```python
from build123d import *

# Parameters (mm, degrees)
BOSS_EXTRUDE1_DEPTH = 3
SKETCH4_W           = 10.2
SKETCH4_H           = 3.2
SKETCH4_W_2         = 3.2
SKETCH4_H_2         = 10.2
SKETCH4_W_3         = 29.422217102
SKETCH4_H_3         = 12.077782898
CUT_EXTRUDE1_DEPTH  = 4


with BuildPart() as part:
    # Sketch1 → Boss-Extrude1 (new body)
    with BuildSketch(Plane(origin=(0, 0, 0), x_dir=(1, 0, 0), z_dir=(0, 1, 0))):
        Polygon((129.394434203, 22.05), (22.05, 22.05), (22.05, 110.344434203), (0, 110.344434203), (0, 0), (129.394434203, 0), align=None)
    extrude(amount=-BOSS_EXTRUDE1_DEPTH)

    # Sketch4 → Cut-Extrude1 (cut, through all)
    with BuildSketch(Plane(origin=(0, 0, 0), x_dir=(1, 0, 0), z_dir=(0, 1, 0))):
        with Locations((54.222217102, 20.55)):
            Rectangle(SKETCH4_W, SKETCH4_H)
        with Locations((74.222217102, 20.55)):
            Rectangle(SKETCH4_W, SKETCH4_H)
        with Locations((114.222217102, 1.5)):
            Rectangle(SKETCH4_W, SKETCH4_H)
        with Locations((1.5, 15.172217102)):
            Rectangle(SKETCH4_W_2, SKETCH4_H_2)
        with Locations((34.222217102, 20.55)):
            Rectangle(SKETCH4_W, SKETCH4_H)
        with Locations((24.611108551, 1.5)):
            Rectangle(SKETCH4_W_3, SKETCH4_H)
        with Locations((32.35, 9.6)):
            Rectangle(SKETCH4_W, SKETCH4_H)
        with Locations((54.222217102, 1.5)):
            Rectangle(SKETCH4_W, SKETCH4_H)
        with Locations((74.222217102, 1.5)):
            Rectangle(SKETCH4_W, SKETCH4_H)
        with Locations((9.6, 15.172217102)):
            Rectangle(SKETCH4_W_2, SKETCH4_H_2)
        with Locations((1.5, 35.172217102)):
            Rectangle(SKETCH4_W_2, SKETCH4_H_2)
        with Locations((9.6, 35.172217102)):
            Rectangle(SKETCH4_W_2, SKETCH4_H_2)
        with Locations((20.55, 35.172217102)):
            Rectangle(SKETCH4_W_2, SKETCH4_H_2)
        with Locations((1.5, 108.844434203)):
            Rectangle(SKETCH4_W_2, SKETCH4_H)
        with Locations((9.6, 108.844434203)):
            Rectangle(SKETCH4_W_2, SKETCH4_H)
        with Locations((9.6, 95.172217102)):
            Rectangle(SKETCH4_W_2, SKETCH4_H_2)
        with Locations((1.5, 95.172217102)):
            Rectangle(SKETCH4_W_2, SKETCH4_H_2)
        with Locations((1.5, 75.172217102)):
            Rectangle(SKETCH4_W_2, SKETCH4_H_2)
        with Locations((9.6, 75.172217102)):
            Rectangle(SKETCH4_W_2, SKETCH4_H_2)
        with Locations((20.55, 95.172217102)):
            Rectangle(SKETCH4_W_2, SKETCH4_H_2)
        with Locations((20.55, 75.172217102)):
            Rectangle(SKETCH4_W_2, SKETCH4_H_2)
        with Locations((1.5, 55.172217102)):
            Rectangle(SKETCH4_W_2, SKETCH4_H_2)
        with Locations((9.6, 55.172217102)):
            Rectangle(SKETCH4_W_2, SKETCH4_H_2)
        with Locations((20.55, 55.172217102)):
            Rectangle(SKETCH4_W_2, SKETCH4_H_2)
        with Locations((127.894434203, 16.111108551)):
            Rectangle(SKETCH4_W_2, SKETCH4_H_3)
        with Locations((94.222217102, 1.5)):
            Rectangle(SKETCH4_W, SKETCH4_H)
        with Locations((114.222217102, 20.55)):
            Rectangle(SKETCH4_W, SKETCH4_H)
        with Locations((94.222217102, 20.55)):
            Rectangle(SKETCH4_W, SKETCH4_H)
        with Locations((116.094434203, 9.6)):
            Rectangle(SKETCH4_W, SKETCH4_H)
    extrude(amount=-CUT_EXTRUDE1_DEPTH, mode=Mode.SUBTRACT)


solid = part.part
```
Can you work these out from the model? Positions are in its coordinate system, mm. A direction names the side the tool comes from. Give positions to 0.01 mm unless a question says otherwise; leave off trailing zeros. Loops run counter-clockwise (first coordinate to the right, second up) from the corner with the lowest first, then second, coordinate; pieces in that order, holes last. Notation, with made-up numbers: M 48.5,12.25 L 54.5,12.25 A8 cw 54.5,16.25 Z; hole C 58,-2 d11. An arc over 180 degrees is marked long. One line per item, written item: value.
(1) We'd pull the mould along X, two halves only. Please class faces 1 (the face through (22.05, -1, -85)), 2 (the face through (9.9, -1, -2)), 3 (the face through (2, -1, -90.072)): released by +X, released by -X, zero draft, split by the parting line, or undercut.
Returned:
face 1: released by +X
face 2: undercut
face 3: zero draft
(2) Suppose I cut it at C-C on y = -1.25. Count the separate pieces of the cut face and the enclosed holes in it, plus the area to 3 significant figures.
Returned:
separate pieces: 1
enclosed holes: 7
area: 3,850 mm^2
(3) Will these pins go through, and if not, where does the flat tip stop? pin 1 (0.9 mm diameter, centred on y = -1, z = -54, fed in from +X); pin 2 (1.5 mm diameter, centred on x = 1.5, y = -1, fed in from -Z); pin 3 (0.9 mm diameter, centred on y = -1, z = -20, fed in from +X).
Returned:
pin 1: x = 18.95
pin 2: z = -107.24
pin 3: x = 126.29
(4) I need wall thicknesses on line 1 (X direction, y = -1.4, z = -21); line 2 (X direction, y = -2.55, z = -95.5); line 3 (Z direction, x = 117, y = -1.25). Which ranges of each line are inside material? Lowest first, please.
Returned:
line 1: 0 to 29.12, 39.32 to 49.12, 59.32 to 69.12, 79.32 to 89.12, 99.32 to 109.12, 119.32 to 126.29
line 2: 3.1 to 8, 11.2 to 18.95
line 3: -18.95 to -11.2, -8 to -3.1
(5) Suppose I cut it at A-A on z = -95. List the corners of the cut face in (x, y) for me.
Returned:
outline: M 3.1,-3 L 8,-3 L 8,0 L 3.1,0 Z; M 11.2,-3 L 18.95,-3 L 18.95,0 L 11.2,0 Z
(6) Which directions (+Z, -Z, +X, -X, +Y, -Y) give clear straight access to the entire face, cutting with the end or side of a thin tool? Please do faces 4 (the face through (109.122, -1, -20)), 5 (the face through (22.05, -1, -26)), 6 (the face through (11.2, -1, -55)), 7 (the face through (119.322, -1, -2)).
Returned:
face 4: -Z, +Y, -Y
face 5: -Z, +X, +Y, -Y
face 6: +Y, -Y
face 7: +Z, +Y, -Y
(7) Suppose I cut it at B-B on x = 15. List the corners of the cut face in (y, z) for me, plus the area to 3 significant figures.
Returned:
outline: M -3,-110.34 L 0,-110.34 L 0,-3.1 L -3,-3.1 Z
area: 322 mm^2
(8) Suppose I cut it at D-D on x = 73.5. List the corners of the cut face in (y, z) for me.
Returned:
outline: M -3,-18.95 L 0,-18.95 L 0,-3.1 L -3,-3.1 Z
